Work out the finished part from the listing and answer in its coordinate system (mm). A direction names the side the tool comes from. Round coordinates to 2 decimals unless told otherwise and drop trailing zeros. Loops run counter-clockwise (first coordinate to the right, second up) from the corner with the lowest first, then second, coordinate; pieces in that order, holes last.
from build123d import *

# Parameters (mm, degrees)
SKETCH1_W           = 40
SKETCH1_H           = 20
BOSS_EXTRUDE1_DEPTH = 9.5
CUT_EXTRUDE1_DEPTH  = 2
FILLET1_START       = -10
FILLET1_DEPTH       = 20
FILLET1_START_2     = -21
FILLET1_2_DEPTH     = 42
SKETCH4_R           = 2.15
CUT_EXTRUDE2_DEPTH  = 30.83705763
SKETCH5_R           = 1.5
SKETCH5_R_2         = 1.65
CUT_EXTRUDE3_DEPTH  = 25.29506135
SKETCH6_R           = 3.5
CUT_EXTRUDE4_DEPTH  = 2


with BuildPart() as part:
    # Sketch1 → Boss-Extrude1 (new body)
    with BuildSketch(Plane.XY):
        Rectangle(SKETCH1_W, SKETCH1_H)
    extrude(amount=BOSS_EXTRUDE1_DEPTH)

    # Sketch3 → Cut-Extrude1 (cut)
    with BuildSketch(Plane(origin=(0, 0, 0), x_dir=(-1, 0, 0), z_dir=(0, 0, -1))):
        with BuildLine():
            Line((13.371397425, -3.45), (1.371397425, -3.45))
            add(Edge.make_bspline(
                [(-6.426606991, -6.332711355), (-3.012827406, -3.55467535), (1.371397425, -3.45)],
                knots=[0, 0, 0, 1, 1, 1], degree=2))
            ThreePointArc((-6.426606991, -6.332711355), (-18.228602575, 0), (-6.426606991, 6.332711355))
            add(Edge.make_bspline(
                [(-6.426606991, 6.332711355), (-3.012827406, 3.55467535), (1.371397425, 3.45)],
                knots=[0, 0, 0, 1, 1, 1], degree=2))
            Line((1.371397425, 3.45), (13.371397425, 3.45))
            ThreePointArc((13.371397425, 3.45), (16.821397425, 0), (13.371397425, -3.45))
        make_face()
    extrude(amount=-CUT_EXTRUDE1_DEPTH, mode=Mode.SUBTRACT)

    # Fillet1: read off the stored shape, not the designer's step
    # Fillet1 outline → Fillet1 (cut)
    with BuildSketch(Plane(origin=(0, 0, 0), x_dir=(1, 0, 0), z_dir=(0, 1, 0)).offset(FILLET1_START)):
        with BuildLine():
            add(Edge.make_bspline(
                [(-20, -1), (-20, 0), (-19, 0)],
                knots=[0, 0, 0, 1, 1, 1], degree=2, weights=[1, 0.707106781, 1]))
            Line((-19, 0), (-20, 0))
            Line((-20, 0), (-20, -1))
        make_face()
        with BuildLine():
            add(Edge.make_bspline(
                [(20, -1), (20, 0), (19, 0)],
                knots=[0, 0, 0, 1, 1, 1], degree=2, weights=[1, 0.707106781, 1]))
            Line((20, -1), (20, 0))
            Line((20, 0), (19, 0))
        make_face()
    extrude(amount=FILLET1_DEPTH, mode=Mode.SUBTRACT)

    # Fillet1 2 outline → Fillet1 2 (cut)
    with BuildSketch(Plane.YZ.offset(FILLET1_START_2)):
        with BuildLine():
            Line((10, 0), (10, 1))
            add(Edge.make_bspline(
                [(10, 1), (10, 0), (9, 0)],
                knots=[0, 0, 0, 1, 1, 1], degree=2, weights=[1, 0.707106781, 1]))
            Line((9, 0), (10, 0))
        make_face()
        with BuildLine():
            Line((-10, 0), (-9, 0))
            add(Edge.make_bspline(
                [(-10, 1), (-10, 0), (-9, 0)],
                knots=[0, 0, 0, 1, 1, 1], degree=2, weights=[1, 0.707106781, 1]))
            Line((-10, 1), (-10, 0))
        make_face()
    extrude(amount=FILLET1_2_DEPTH, mode=Mode.SUBTRACT)

    # Sketch4 → Cut-Extrude2 (cut, through all)
    with BuildSketch(Plane(origin=(0, 10, 0), x_dir=(1, 0, 0), z_dir=(0, 1, 0))):
        with Locations(Location((-15.5, -4.8, 0), (0, 0, 180))):
            Circle(SKETCH4_R)
        with Locations(Location((-5.5, -4.8, 0), (0, 0, 180))):
            Circle(SKETCH4_R)
        with Locations(Location((5.63, -4.8, 0), (0, 0, 180))):
            Circle(SKETCH4_R)
        with Locations(Location((15.63, -4.8, 0), (0, 0, 180))):
            Circle(SKETCH4_R)
    extrude(amount=-CUT_EXTRUDE2_DEPTH, mode=Mode.SUBTRACT)

    # Sketch5 → Cut-Extrude3 (cut, through all)
    with BuildSketch(Plane(origin=(0, 0, 0), x_dir=(-1, 0, 0), z_dir=(0, 0, -1))):
        with Locations((13.371397425, 0)):
            Circle(SKETCH5_R)
        with Locations((9.371397425, 0)):
            Circle(SKETCH5_R_2)
        with Locations((-10.628602575, 0)):
            Circle(SKETCH5_R_2)
    extrude(amount=-CUT_EXTRUDE3_DEPTH, mode=Mode.SUBTRACT)

    # Sketch6 → Cut-Extrude4 (cut)
    with BuildSketch(Plane.XY.offset(9.5)):
        with Locations((10.628602575, 0)):
            Circle(SKETCH6_R)
        with Locations((-9.371397425, 0)):
            Circle(SKETCH6_R)
    extrude(amount=-CUT_EXTRUDE4_DEPTH, mode=Mode.SUBTRACT)


solid = part.part
Item 1: Section A-A, the plane z = 6 is taken. Give the vertices of the cut face in (x, y).
Item 2: Section B-B, the plane y = 0 is taken. State how many separate pieces and enclosed holes the cut face has, plus the area to 3 significant figures.
Item 3: For faces 1 (the face through (-7, 3.45, 1)), 2 (the face through (11, -2, 7.5)), 3 (the face through (0, 10, 5)), determine the directions among +Z, -Z, +X, -X, +Y, -Y from which every point of the face is accessible in a straight line to the end or side of a thin tool.
Item 4: Each of these flat-tipped pins is pushed along its axis until it touches: P1, Ø4.5, axis at x = 10.63, y = 0, coming from the +Z side; P2, Ø4.5, axis at x = -9.37, y = 0, coming from the -Z side. Where does it stop, or does it pass through?
Item 5: Straight lines are drawn through the part: line 1 (Y direction, x = 10.5, z = 6); line 2 (Z direction, x = -15.5, y = 4.5); line 3 (X direction, y = -5.75, z = 3.5). For each, find the intervals that lie inside material, in ascending order.
Item 6: Determine the mould class of faces 4 (the face through (0, -10, 5)), 5 (the face through (0, 0, 9.5)), 6 (the face through (18.225, -0.229, 0.986)) for opening direction Y: pulls with the +Y half, pulls with the -Y half, needs draft (parallel to the pull), parting line crosses it, or undercut.
Item 7: Section C-C, the plane z = 4.25 is taken. Give the vertices of the cut face in (x, y).
Answer below:
1. outline: (-20, -10) - (-17.28, -10) - (-17.28, 10) - (-20, 10) - close; (-13.72, -10) - (-7.28, -10) - (-7.28, 10) - (-13.72, 10) - (-13.72, 1.46) arc R1.5 cw (long way) to (-13.72, -1.46) - close; (-3.72, -10) - (3.85, -10) - (3.85, 10) - (-3.72, 10) - close; (7.41, -10) - (13.85, -10) - (13.85, 10) - (7.41, 10) - close; (17.41, -10) - (20, -10) - (20, 10) - (17.41, 10) - close; hole circle Ø3.3 at (-9.37, 0); hole circle Ø3.3 at (10.63, 0)
2. separate pieces: 4
2. enclosed holes: 3
2. area: 171 mm2
3. face 1: -Z
3. face 2: +Z
3. face 3: +Z, -Z, +X, -X, +Y
4. P1: stops at z = 7.5
4. P2: stops at z = 2
5. line 1: y = -10 to -1.64, 1.64 to 10
5. line 2: z = 0 to 2.65, 6.95 to 9.5
5. line 3: x = -20 to -17.21, -13.79 to -7.21, -3.79 to 3.92, 7.34 to 13.92, 17.34 to 20
6. face 4: pulls with the -Y half
6. face 5: needs draft
6. face 6: undercut
7. outline: (-20, -10) - (-17.58, -10) - (-17.58, 10) - (-20, 10) - close; (-13.42, -10) - (-7.58, -10) - (-7.58, 10) - (-13.42, 10) - (-13.42, 1.5) arc R1.5 cw (long way) to (-13.42, -1.5) - close; (-3.42, -10) - (3.55, -10) - (3.55, 10) - (-3.42, 10) - close; (7.71, -10) - (13.55, -10) - (13.55, 10) - (7.71, 10) - close; (17.71, -10) - (20, -10) - (20, 10) - (17.71, 10) - close; hole circle Ø3.3 at (-9.37, 0); hole circle Ø3.3 at (10.63, 0)
